The model under review builds one solid part; all positions refer to its coordinate system, in mm. Face numbers are marked on the shaded views. Coordinates: 2 decimals unless noted, no trailing zeros. Order: outer loops, then holes, each group sorted by start corner. A loop starts at its lowest first (then second) coordinate and runs counter-clockwise, first axis right, second up. Notation, with made-up numbers: (9, 3) - (30, 3) arc R26 ccw to (30, 18) - close; hole circle Ø1 at (33, 22). An arc over 180 degrees is marked (long way). Answer in a Markdown table with one row per item.
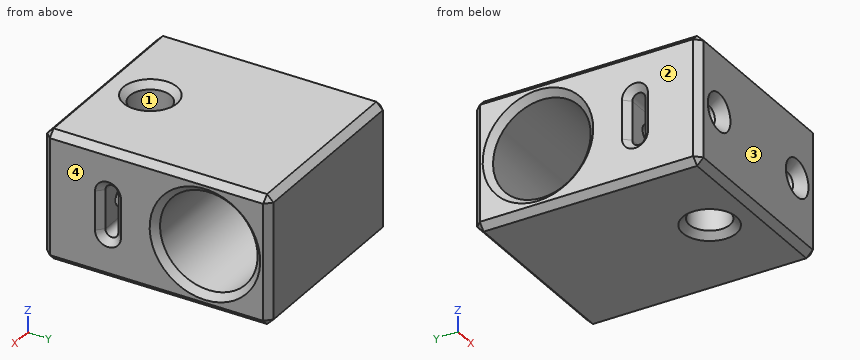
```python
from build123d import *

# Parameters (mm, degrees)
SKETCH_1_W          = 20
SKETCH_1_H          = 35
SKETCH_1_R          = 7.55
EXTRUDE_1_DEPTH     = 30
CUT_EXTRUDE_1_REACH = 22
SKETCH_2_R          = 3.15
CUT_EXTRUDE_2_DEPTH = 10
CUT_EXTRUDE_3_DEPTH = 10
SKETCH_5_R          = 1.4
CUT_EXTRUDE_4_DEPTH = 13
CHAMFER_1_SIZE      = 1
CHAMFER_2_SIZE      = 1.5


with BuildPart() as part:
    # 草图1 → 凸台-拉伸1 (new body)
    with BuildSketch(Plane(origin=(0, 0, 0), x_dir=(0, 0, -1), z_dir=(1, 0, 0))):
        with Locations((10, 17.5)):
            Rectangle(SKETCH_1_W, SKETCH_1_H)
        with Locations((10, 25)):
            Circle(SKETCH_1_R, mode=Mode.SUBTRACT)
    extrude(amount=EXTRUDE_1_DEPTH)

    # 草图2 → 切除-拉伸1 (cut, up to next)
    with BuildSketch(Plane.XY, mode=Mode.PRIVATE) as cut_extrude_1_sk1:
        with Locations((15, 7.5)):
            Circle(SKETCH_2_R)
    cut_extrude_1_tool1 = extrude(cut_extrude_1_sk1.sketch, amount=-CUT_EXTRUDE_1_REACH, mode=Mode.PRIVATE) & part.part
    add(cut_extrude_1_tool1.solids().sort_by_distance((15, 7.5, 0))[0], mode=Mode.SUBTRACT)

    # 草图3 → 切除-拉伸2 (cut)
    with BuildSketch(Plane(origin=(30, 0, 0), x_dir=(0, 0, -1), z_dir=(1, 0, 0))):
        with BuildLine():
            Line((7, 11), (13, 11))
            ThreePointArc((13, 11), (14, 10), (13, 9))
            Line((13, 9), (7, 9))
            ThreePointArc((7, 9), (6, 10), (7, 11))
        make_face()
    extrude(amount=-CUT_EXTRUDE_2_DEPTH, mode=Mode.SUBTRACT)

    # 草图4 → 切除-拉伸3 (cut)
    with BuildSketch(Plane.ZY):
        with BuildLine():
            Line((-7, 9), (-13, 9))
            ThreePointArc((-13, 9), (-14, 10), (-13, 11))
            Line((-13, 11), (-7, 11))
            ThreePointArc((-7, 11), (-6, 10), (-7, 9))
        make_face()
    extrude(amount=-CUT_EXTRUDE_3_DEPTH, mode=Mode.SUBTRACT)

    # 草图5 → 切除-拉伸4 (cut)
    with BuildSketch(Plane.XZ):
        with Locations((5, -10)):
            Circle(SKETCH_5_R)
        with Locations((25, -10)):
            Circle(SKETCH_5_R)
    extrude(amount=-CUT_EXTRUDE_4_DEPTH, mode=Mode.SUBTRACT)

    # 倒角1
    chamfer_1_edges = [part.edges().sort_by_distance(p)[0] for p in [
        (0, 25, -2.45),
        (30, 25, -2.45),
        (30, 35, -10),
        (30, 17.5, 0),
        (11.85, 7.5, 0),
        (11.85, 7.5, -20),
        (30, 10, -6),
        (30, 9, -10),
        (30, 10, -14),
        (30, 11, -10),
        (0, 10, -6),
        (0, 11, -10),
        (0, 10, -14),
        (0, 9, -10),
        (30, 0, -10),
        (0, 17.5, 0),
        (0, 35, -10),
        (0, 17.5, -20),
        (0, 0, -10),
        (15, 0, 0),
        (15, 35, 0),
        (15, 35, -20),
        (15, 0, -20),
        (30, 17.5, -20),
    ]]
    chamfer(chamfer_1_edges, length=CHAMFER_1_SIZE)

    # 倒角2
    chamfer_2_edges = [part.edges().sort_by_distance(p)[0] for p in [
        (3.6, 0, -10),
        (23.6, 0, -10),
    ]]
    chamfer(chamfer_2_edges, length=CHAMFER_2_SIZE)


solid = part.part
```
Item 1: Mouldability with a two-part tool opening along X and no side actions: class the marked faces 1, 2, 3 and 4 as +X half, -X half, draft (parallel to the pull), parting line (faces both ways), or undercut.
Check values:
| item | result |
|---|---|
| face 1 | undercut |
| face 2 | -X half |
| face 3 | draft |
| face 4 | +X half |
Item 2: We need section A-A, the plane y = 7.5. Write out the cut boundary in (x, z), then the cut area to 3 significant figures.
Check values:
| item | result |
|---|---|
| outline | (0, -19) - (1, -20) - (10.85, -20) - (11.85, -19) - (11.85, -1) - (10.85, 0) - (1, 0) - (0, -1) - close; (18.15, -19) - (19.15, -20) - (29, -20) - (30, -19) - (30, -1) - (29, 0) - (19.15, 0) - (18.15, -1) - close; hole circle Ø2.8 at (5, -10); hole circle Ø2.8 at (25, -10) |
| area | 458 mm^2 |
Item 3: We need section B-B, the plane x = 5. Write out the cut boundary in (y, z), then the cut area to 3 significant figures.
Check values:
| item | result |
|---|---|
| outline | (0, -19) - (1, -20) - (34, -20) - (35, -19) - (35, -1) - (34, 0) - (1, 0) - (0, -1) - (0, -7.1) - (1.5, -8.6) - (9, -8.6) - (9, -7) arc R1 cw to (11, -7) - (11, -8.6) - (13, -8.6) - (13, -11.4) - (11, -11.4) - (11, -13) arc R1 cw to (9, -13) - (9, -11.4) - (1.5, -11.4) - (0, -12.9) - close; hole circle Ø15.1 at (25, -10) |
| area | 471 mm^2 |
Item 4: We need section C-C, the plane z = -10.5. State how many separate pieces and enclosed holes the cut face has, then the cut area to 3 significant figures.
Check values:
| item | result |
|---|---|
| separate pieces | 4 |
| enclosed holes | 1 |
| area | 459 mm^2 |
Item 5: To check wall thickness, follow line 1 (Y direction, x = 7, z = -10); line 2 (Y direction, x = 10.5, z = -10); line 3 (Y direction, x = 15.75, z = -7.25). State the ranges of each line that lie inside material, in increasing order. Write a range as from..to.
Check values:
| item | result |
|---|---|
| line 1 | 0.9..9, 11..17.45, 32.55..35 |
| line 2 | 0..17.45, 32.55..35 |
| line 3 | 0..4.44, 10.56..17.97, 32.03..35 |
Item 6: Clearance check with flat-ended pins moving along their axes: pin 1 Ø4.5 at (x, z) = (5, -10) entering from -Y; pin 2 Ø1.5 at (y, z) = (17, -14.5) entering from -X; pin 3 Ø2 at (y, z) = (9.5, -10) entering from +X; pin 4 Ø5 at (x, y) = (15, 7.5) entering from -Z. State where each tip first meets the part, or that it passes through.
Check values:
| item | result |
|---|---|
| pin 1 | y = 0.65 |
| pin 2 | x = 0 |
| pin 3 | x = 29.5 |
| pin 4 | through |
